from build123d import *

# Parameters (mm, degrees)
SKETCH1_W               = 62.4208
SKETCH1_H               = 60
SKETCH1_R               = 13.5
BOSS_EXTRUDE1_DEPTH     = 1.8
BOSS_EXTRUDE2_START     = -1.8
SKETCH2_W               = 53.9308
SKETCH2_H               = 4.6
BOSS_EXTRUDE2_DEPTH     = 7
BOSS_EXTRUDE3_DEPTH     = 8.5
CUT_EXTRUDE1_REACH      = 72.058
CUT_EXTRUDE1_END_RADIUS = 39.6875
SKETCH4_R               = 2.5


with BuildPart() as part:
    # Sketch1 → Boss-Extrude1 (new body)
    with BuildSketch(Plane.XY):
        with Locations((6.283906244, 0.094262462)):
            Rectangle(SKETCH1_W, SKETCH1_H)
        with Locations((15.494306244, 0.094262462)):
            Circle(SKETCH1_R, mode=Mode.SUBTRACT)
    extrude(amount=BOSS_EXTRUDE1_DEPTH)

    # Sketch2 → Boss-Extrude2 (add)
    with BuildSketch(Plane.XY.offset(1.8).offset(BOSS_EXTRUDE2_START)):
        with Locations((2.038906244, -27.605737538)):
            Rectangle(SKETCH2_W, SKETCH2_H)
        with Locations((2.038906244, 27.794262462)):
            Rectangle(SKETCH2_W, SKETCH2_H)
    extrude(amount=-BOSS_EXTRUDE2_DEPTH)

    # Sketch3 → Boss-Extrude3 (add)
    with BuildSketch(Plane.XY.offset(1.8)):
        with BuildLine():
            ThreePointArc((-10.488335197, -29.905737538), (-19.588138729, -18.461591357), (-23.926493756, -4.49901345))
            ThreePointArc((-23.926493756, -4.49901345), (-24.193193756, 0.094262462), (-23.926493756, 4.687538375))
            ThreePointArc((-23.926493756, 4.687538375), (-19.588138729, 18.650116281), (-10.488335197, 30.094262462))
            Line((-10.488335197, 30.094262462), (-24.926493756, 30.094262462))
            Line((-24.926493756, 30.094262462), (-24.926493756, -29.905737538))
            Line((-24.926493756, -29.905737538), (-10.488335197, -29.905737538))
        make_face()
    extrude(amount=BOSS_EXTRUDE3_DEPTH)

    # Cut-Extrude1: up to this cylinder (the profile starts outside it)
    cut_extrude1_end = Plane(origin=(15.494306244, 0.094262462, 6.499), z_dir=(0, 0, -1)) * Cylinder(CUT_EXTRUDE1_END_RADIUS, 224.491, mode=Mode.PRIVATE)
    # Sketch4 → Cut-Extrude1 (cut, up to the surface)
    with BuildSketch(Plane.ZY.offset(24.926493756), mode=Mode.PRIVATE) as cut_extrude1_sk1:
        with Locations((6.499, 0.094262462)):
            Circle(SKETCH4_R)
    cut_extrude1_tool1 = extrude(cut_extrude1_sk1.sketch, amount=-CUT_EXTRUDE1_REACH, mode=Mode.PRIVATE) - cut_extrude1_end
    add(cut_extrude1_tool1.solids().sort_by_distance((-24.926494, 0.094262, 6.499))[0], mode=Mode.SUBTRACT)


solid = part.part
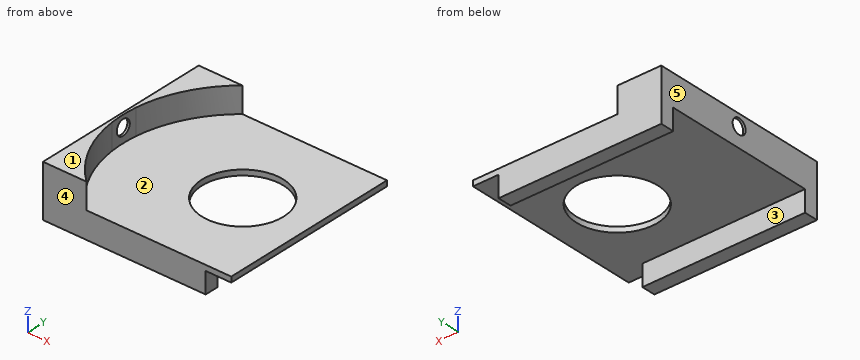
For this review, take the finished solid that the model builds, in its own axes (mm). Face numbers are marked on the shaded views. A direction names the side the tool comes from. Round coordinates to 2 decimals unless told otherwise and drop trailing zeros. Write each loop counter-clockwise with the first axis right and the second up, starting at its lowest first coordinate (ties: lowest second). Pieces come first, ordered by that corner, then holes. Notation, with made-up numbers: (9.25, -26) -> (45.25, -26) arc R20 cw to (45.25, 3) -> close; hole circle Ø8 at (-17.5, 13). An arc over 180 degrees is marked (long way). Put each result on its own line as item: value.
Q1. Clearance check with flat-ended pins moving along their axes: pin 1 Ø24.5 at (x, y) = (15.49, 0.09) entering from +Z; pin 2 Ø1.4 at (y, z) = (-26.5, -3.5) entering from +X; pin 3 Ø18 at (x, y) = (0.5, 1) entering from -Z; pin 4 Ø1.5 at (x, y) = (-10.5, 19.5) entering from +Z. State where each tip first meets the part, or that it passes through.
Determined:
pin 1: passes through
pin 2: stops at x = 29
pin 3: stops at z = 0
pin 4: stops at z = 1.8
Q2. Consider section B-B on x = 25. State the section outline as (y, z) points.
Determined:
outline: (-29.91, -7) -> (-25.31, -7) -> (-25.31, 0) -> (-9.49, 0) -> (-9.49, 1.8) -> (-29.91, 1.8) -> close; (9.68, 0) -> (25.49, 0) -> (25.49, -7) -> (30.09, -7) -> (30.09, 1.8) -> (9.68, 1.8) -> close
Q3. To check wall thickness, follow L1, parallel to Y at x = 14.5, z = -2.5; L2, parallel to Z at x = 32, y = -27; L3, parallel to Z at x = -9, y = 26. State the ranges of each line that lie inside material, in increasing order. Write a range as [from, to].
Determined:
L1: y = [-29.91, -25.31], [25.49, 30.09]
L2: z = [0, 1.8]
L3: z = [-7, 1.8]
Q4. Consider section A-A on z = -1. State the section outline as (x, y) points.
Determined:
outline: (-24.93, -29.91) -> (29, -29.91) -> (29, -25.31) -> (-24.93, -25.31) -> close; (-24.93, 25.49) -> (29, 25.49) -> (29, 30.09) -> (-24.93, 30.09) -> close
Q5. The part is to be moulded in two halves that separate along Y. For the marked faces 3, 4 and 5, say which applies: released by +Y, released by -Y, zero draft, split by the parting line, or undercut.
Determined:
face 3: undercut
face 4: released by -Y
face 5: zero draft
Q6. Consider section D-D on x = -3.5. State the section outline as (y, z) points, and give its area (3 significant figures).
Determined:
outline: (-29.91, -7) -> (-25.31, -7) -> (-25.31, 0) -> (25.49, 0) -> (25.49, -7) -> (30.09, -7) -> (30.09, 1.8) -> (-29.91, 1.8) -> close
area: 172 mm^2
Q7. Machinability: for the marked faces 1 and 2, which of the approach directions +Z, -Z, +X, -X, +Y, -Y give a long, thin tool a straight path to every point of the face, cutting with its end or side? Answer none if there is none.
Determined:
face 1: +Z, +X, -X, +Y, -Y
face 2: +Z, +X
Q8. Consider section C-C on y = 6. State the section outline as (x, z) points.
Determined:
outline: (-24.93, 0) -> (3.35, 0) -> (3.35, 1.8) -> (-23.75, 1.8) -> (-23.75, 10.3) -> (-24.93, 10.3) -> close; (27.63, 0) -> (37.49, 0) -> (37.49, 1.8) -> (27.63, 1.8) -> close
